from build123d import *

# Parameters (mm, degrees)
SKETCH1_R           = 1.75
BOSS_EXTRUDE1_DEPTH = 4
SKETCH2_R           = 1.3
SKETCH2_R_2         = 2.4
CUT_EXTRUDE1_DEPTH  = 38.915688046


with BuildPart() as part:
    # Sketch1 → Boss-Extrude1 (new body)
    with BuildSketch(Plane.XY):
        with BuildLine():
            ThreePointArc((30.75, -4), (34.75, 0), (30.75, 4))
            Line((30.75, 4), (14.072558403, 4))
            ThreePointArc((14.072558403, 4), (14.06038767, 4.04257326), (14.048088143, 4.085109489))
            ThreePointArc((14.048088143, 4.085109489), (12.712915648, 4.255390909), (11.377106712, 4.090176385))
            ThreePointArc((11.377106712, 4.090176385), (11.169703548, 4.626642697), (10.937020765, 5.152637848))
            ThreePointArc((10.937020765, 5.152637848), (11.998404632, 5.980373095), (12.82210701, 7.044889767))
            ThreePointArc((12.82210701, 7.044889767), (12.669951657, 7.315), (12.51210701, 7.581825517))
            ThreePointArc((12.51210701, 7.581825517), (11.17835734, 7.400736668), (9.930825655, 6.8954189))
            ThreePointArc((9.930825655, 6.8954189), (9.591641884, 7.359925677), (9.230750012, 7.807775241))
            ThreePointArc((9.230750012, 7.807775241), (10.041734454, 8.882012453), (10.561852666, 10.123446462))
            ThreePointArc((10.561852666, 10.123446462), (10.344972209, 10.344972209), (10.123446462, 10.561852666))
            ThreePointArc((10.123446462, 10.561852666), (8.882012453, 10.041734454), (7.807775241, 9.230750012))
            ThreePointArc((7.807775241, 9.230750012), (7.359925677, 9.591641884), (6.8954189, 9.930825655))
            ThreePointArc((6.8954189, 9.930825655), (7.400736668, 11.17835734), (7.581825517, 12.51210701))
            ThreePointArc((7.581825517, 12.51210701), (7.315, 12.669951657), (7.044889767, 12.82210701))
            ThreePointArc((7.044889767, 12.82210701), (5.980373095, 11.998404632), (5.152637848, 10.937020765))
            ThreePointArc((5.152637848, 10.937020765), (4.626642697, 11.169703548), (4.090176385, 11.377106712))
            ThreePointArc((4.090176385, 11.377106712), (4.255390909, 12.712915648), (4.085109489, 14.048088143))
            ThreePointArc((4.085109489, 14.048088143), (3.78652263, 14.131494839), (3.486235477, 14.208555951))
            ThreePointArc((3.486235477, 14.208555951), (2.671181194, 13.137403362), (2.1463567, 11.897951627))
            ThreePointArc((2.1463567, 11.897951627), (1.578061664, 11.986568374), (1.00619511, 12.048056748))
            ThreePointArc((1.00619511, 12.048056748), (0.820047291, 13.381109763), (0.31, 14.626715284))
            ThreePointArc((0.31, 14.626715284), (0, 14.63), (-0.31, 14.626715284))
            ThreePointArc((-0.31, 14.626715284), (-0.820047291, 13.381109763), (-1.00619511, 12.048056748))
            ThreePointArc((-1.00619511, 12.048056748), (-1.578061664, 11.986568374), (-2.1463567, 11.897951627))
            ThreePointArc((-2.1463567, 11.897951627), (-2.671181194, 13.137403362), (-3.486235477, 14.208555951))
            ThreePointArc((-3.486235477, 14.208555951), (-3.78652263, 14.131494839), (-4.085109489, 14.048088143))
            ThreePointArc((-4.085109489, 14.048088143), (-4.255390909, 12.712915648), (-4.090176385, 11.377106712))
            ThreePointArc((-4.090176385, 11.377106712), (-4.626642697, 11.169703548), (-5.152637848, 10.937020765))
            ThreePointArc((-5.152637848, 10.937020765), (-5.980373095, 11.998404632), (-7.044889767, 12.82210701))
            ThreePointArc((-7.044889767, 12.82210701), (-7.315, 12.669951657), (-7.581825517, 12.51210701))
            ThreePointArc((-7.581825517, 12.51210701), (-7.400736668, 11.17835734), (-6.8954189, 9.930825655))
            ThreePointArc((-6.8954189, 9.930825655), (-7.359925677, 9.591641884), (-7.807775241, 9.230750012))
            ThreePointArc((-7.807775241, 9.230750012), (-8.882012453, 10.041734454), (-10.123446462, 10.561852666))
            ThreePointArc((-10.123446462, 10.561852666), (-10.344972209, 10.344972209), (-10.561852666, 10.123446462))
            ThreePointArc((-10.561852666, 10.123446462), (-10.041734454, 8.882012453), (-9.230750012, 7.807775241))
            ThreePointArc((-9.230750012, 7.807775241), (-9.591641884, 7.359925677), (-9.930825655, 6.8954189))
            ThreePointArc((-9.930825655, 6.8954189), (-11.17835734, 7.400736668), (-12.51210701, 7.581825517))
            ThreePointArc((-12.51210701, 7.581825517), (-12.669951657, 7.315), (-12.82210701, 7.044889767))
            ThreePointArc((-12.82210701, 7.044889767), (-11.998404632, 5.980373095), (-10.937020765, 5.152637848))
            ThreePointArc((-10.937020765, 5.152637848), (-11.169703548, 4.626642697), (-11.377106712, 4.090176385))
            ThreePointArc((-11.377106712, 4.090176385), (-12.712915648, 4.255390909), (-14.048088143, 4.085109489))
            ThreePointArc((-14.048088143, 4.085109489), (-14.131494839, 3.78652263), (-14.208555951, 3.486235477))
            ThreePointArc((-14.208555951, 3.486235477), (-13.137403362, 2.671181194), (-11.897951627, 2.1463567))
            ThreePointArc((-11.897951627, 2.1463567), (-11.986568374, 1.578061664), (-12.048056748, 1.00619511))
            ThreePointArc((-12.048056748, 1.00619511), (-13.381109763, 0.820047291), (-14.626715284, 0.31))
            ThreePointArc((-14.626715284, 0.31), (-14.63, 0), (-14.626715284, -0.31))
            ThreePointArc((-14.626715284, -0.31), (-13.381109763, -0.820047291), (-12.048056748, -1.00619511))
            ThreePointArc((-12.048056748, -1.00619511), (-11.986568374, -1.578061664), (-11.897951627, -2.1463567))
            ThreePointArc((-11.897951627, -2.1463567), (-13.137403362, -2.671181194), (-14.208555951, -3.486235477))
            ThreePointArc((-14.208555951, -3.486235477), (-14.131494839, -3.78652263), (-14.048088143, -4.085109489))
            ThreePointArc((-14.048088143, -4.085109489), (-12.712915648, -4.255390909), (-11.377106712, -4.090176385))
            ThreePointArc((-11.377106712, -4.090176385), (0.047845736, -12.089905326), (11.409123542, -4))
            Line((11.409123542, -4), (30.75, -4))
        make_face()
        Circle(SKETCH1_R, mode=Mode.SUBTRACT)
        with Locations((30.75, 0)):
            Circle(SKETCH1_R, mode=Mode.SUBTRACT)
    extrude(amount=BOSS_EXTRUDE1_DEPTH)

    # Sketch2 → Cut-Extrude1 (cut, through all)
    with BuildSketch(Plane.XY.offset(4)):
        with Locations((4.5, 0)):
            Circle(SKETCH2_R)
        with Locations((-4.5, 0)):
            Circle(SKETCH2_R)
        Circle(SKETCH2_R_2)
    extrude(amount=-CUT_EXTRUDE1_DEPTH, mode=Mode.SUBTRACT)


solid = part.part
CAD build for the part. Positions are in the model's coordinates, mm. A direction names the side the tool comes from. Give positions to 0.01 mm unless a question says otherwise; leave off trailing zeros. Order: outer loops, then holes, each group sorted by start corner. A loop starts at its lowest first (then second) coordinate and runs counter-clockwise, first axis right, second up. Notation, with made-up numbers: (32, 82) -> (66, 82) arc R37 ccw to (66, 118) -> close; hole circle Ø1 at (3.5, 77.5). An arc over 180 degrees is marked (long way). Return JSON: item names as keys, results as strings.
Q1. Saw through at B-B (x = 15.5). Write the cut outline in (y, z), then the cut area to 3 significant figures.
Working result:
{"outline": "(-4, 0) -> (4, 0) -> (4, 4) -> (-4, 4) -> close", "area": "32.0 mm²"}
Q2. Drill centre lines: line 1 (X direction, y = 13, z = 2); line 2 (Y direction, x = 0, z = 2.85); line 3 (Y direction, x = 30.75, z = 1.25). Where is each one in solid material? Low to high.
Working result:
{"line 1": "-4.25 to -2.59, -0.91 to 0.91, 2.59 to 4.25", "line 2": "-12.09 to -2.4, 2.4 to 14.63", "line 3": "-4 to -1.75, 1.75 to 4"}
Q3. Flat gauge pins, fed straight in: pin 1 (2 mm diameter, centred on y = 11.5, z = 1.5, fed in from -X); pin 2 (1 mm diameter, centred on x = 29.5, z = 3, fed in from +Y). Where does each tip first touch, or does it go through?
Working result:
{"pin 1": "x = -10.19", "pin 2": "y = 4"}
Q4. Saw through at A-A (z = 2.2). Count the separate pieces of the cut face and the enclosed holes in it, then the cut area to 3 significant figures.
Working result:
{"separate pieces": "1", "enclosed holes": "4", "area": "645 mm²"}
Q5. Which spindle directions (+Z, -Z, +X, -X, +Y, -Y) get a long thin tool onto all of the face, cutting with end or side? Do faces 1 (the face through (-11.988, -1.57, 1.972)), 2 (the face through (0.825, 13.363, 1.972)), 3 (the face through (7.366, 9.587, 1.972)). Say none if no direction does.
Working result:
{"face 1": "+Z, -Z, -X", "face 2": "+Z, -Z, +Y", "face 3": "+Z, -Z"}
Q6. Mould opens along X. For faces 4 (the face through (-13.15, 2.68, 1.97)), 5 (the face through (-12.732, -4.255, 1.972)), 6 (the face through (4.2, 1.5, 0)), 7 (the face through (4.255, 12.694, 1.972)) say: pulls with the +X half, pulls with the -X half, needs draft (parallel to the pull), parting line crosses it, or undercut.
Working result:
{"face 4": "pulls with the -X half", "face 5": "undercut", "face 6": "needs draft", "face 7": "undercut"}
